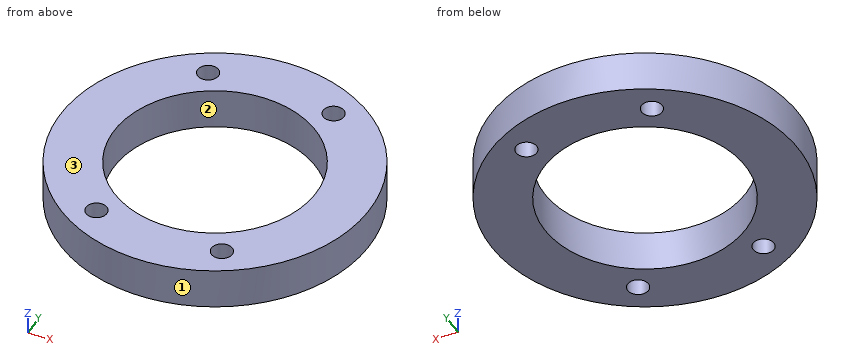
```python
from build123d import *

# Parameters (mm, degrees)
F0_R     = 70.485
F0_R_2   = 4.7625
F0_R_3   = 46.0375
F1_DEPTH = 19.05


with BuildPart() as f1:
    # F0 (on Top) → F1 (new body)
    with BuildSketch(Plane.XY):
        with Locations((-6.82183, 127.916229)):
            Circle(F0_R)
        with Locations((-35.71433, 77.872946)):
            Circle(F0_R_2, mode=Mode.SUBTRACT)
        with Locations((-35.71433, 177.959512)):
            Circle(F0_R_2, mode=Mode.SUBTRACT)
        with Locations((22.07067, 77.872946)):
            Circle(F0_R_2, mode=Mode.SUBTRACT)
        with Locations((-6.82183, 127.916229)):
            Circle(F0_R_3, mode=Mode.SUBTRACT)
        with Locations((22.07067, 177.959512)):
            Circle(F0_R_2, mode=Mode.SUBTRACT)
    extrude(amount=-F1_DEPTH)


solid = f1.part
```
The model under review builds one solid part; all positions refer to its coordinate system, in mm. Face numbers are marked on the shaded views. Round coordinates to 2 decimals unless told otherwise and drop trailing zeros. Loops run counter-clockwise (first coordinate to the right, second up) from the corner with the lowest first, then second, coordinate; pieces in that order, holes last. Notation, with made-up numbers: (49.5, 26.25) - (74.5, 26.25) arc R24 ccw to (74.5, 54.25) - close; hole circle Ø3 at (-3.5, 16.5). An arc over 180 degrees is marked (long way). Write each question's results on one line, items separated by ' | '. Start each with the question number.
Q1. Draft analysis for pull direction X (two halves, no side actions). For the marked faces 1, 2 and 3, state which applies: pulls with the +X half, pulls with the -X half, needs draft (parallel to the pull), parting line crosses it, or undercut.
Q2. Take a section at A-A on y = 107. Give the boundary of the cut face in (x, z).
Q3. Wall thickness on line 1 along X through (y, z) = (80, -13); line 2 along X through (y, z) = (78, -16); line 3 along Y through (x, z) = (21.5, -2.5): over which ranges is each line inside the solid? List them lowest first. Write a range as [from, to].
Q4. Take a section at C-C on z = -10.25. Give the boundary of the cut face in (x, y) (1 decimal).
Q5. Take a section at B-B on y = 90. Give the boundary of the cut face in (x, z).
Q6. Insertion check: P1, Ø12.5, axis at x = 22.07, y = 177.96, coming from the +Z side; P2, Ø8, axis at x = 46, z = -14, coming from the +Y side; P3, Ø2, axis at y = 82, z = -13.5, coming from the +X side; P4, Ø8, axis at x = -8, z = -12.5, coming from the +Y side. Each pin has a flat end and moves straight along its axis. Give the tip position at first contact, or say it passes through.
Q7. Take a section at D-D on x = 52.5. Give the boundary of the cut face in (y, z).
Data:
1) face 1: parting line crosses it | face 2: undercut | face 3: needs draft
2) outline: (-74.13, -19.05) - (-47.83, -19.05) - (-47.83, 0) - (-74.13, 0) - close; (34.19, -19.05) - (60.49, -19.05) - (60.49, 0) - (34.19, 0) - close
3) line 1: x = [-58.51, -39.98], [-31.45, 17.81], [26.33, 44.87] | line 2: x = [-56.59, -40.48], [-30.95, 17.31], [26.83, 42.94] | line 3: y = [63.37, 73.14], [82.6, 91.62], [164.21, 173.23], [182.69, 192.46]
4) outline: circle Ø141 at (-6.8, 127.9); hole circle Ø92.1 at (-6.8, 127.9); hole circle Ø9.5 at (-35.7, 77.9); hole circle Ø9.5 at (-35.7, 178); hole circle Ø9.5 at (22.1, 77.9); hole circle Ø9.5 at (22.1, 178)
5) outline: (-66.24, -19.05) - (-32.93, -19.05) - (-32.93, 0) - (-66.24, 0) - close; (19.29, -19.05) - (52.6, -19.05) - (52.6, 0) - (19.29, 0) - close
6) P1: stops at z = 0 | P2: stops at y = 178.75 | P3: stops at x = 47.5 | P4: stops at y = 198.4
7) outline: (89.85, -19.05) - (165.98, -19.05) - (165.98, 0) - (89.85, 0) - close
